```python
from build123d import *

# Parameters (mm, degrees)
SKETCH1_R           = 3.0607
BOSS_EXTRUDE1_DEPTH = 6.35
SKETCH2_R           = 8.20039
CUT_EXTRUDE1_DEPTH  = 7.35
BOSS_EXTRUDE2_DEPTH = 19.05
SKETCH4_R           = 8.20039
CUT_EXTRUDE2_DEPTH  = 19.05
CUT_EXTRUDE2_TAPER  = -12
SKETCH5_R           = 1.5875
CUT_EXTRUDE3_DEPTH  = 7.35
BOSS_EXTRUDE3_DEPTH = 6.35


with BuildPart() as part:
    # Sketch1 → Boss-Extrude1 (new body)
    with BuildSketch(Plane(origin=(0, 91.487983019, 0), x_dir=(1, 0, 0), z_dir=(0, 1, 0))):
        with BuildLine():
            Line((-19.645108088, -156.928503968), (88.304891912, -156.928503968))
            ThreePointArc((88.304891912, -156.928503968), (95.040084003, -154.138696059), (97.829891912, -147.403503968))
            Line((97.829891912, -147.403503968), (97.829891912, -64.853503968))
            ThreePointArc((97.829891912, -64.853503968), (95.040084003, -58.118311877), (88.304891912, -55.328503968))
            Line((88.304891912, -55.328503968), (-19.645108088, -55.328503968))
            ThreePointArc((-19.645108088, -55.328503968), (-26.380300179, -58.118311877), (-29.170108088, -64.853503968))
            Line((-29.170108088, -64.853503968), (-29.170108088, -147.403503968))
            ThreePointArc((-29.170108088, -147.403503968), (-26.380300179, -154.138696059), (-19.645108088, -156.928503968))
        make_face()
        with Locations((-23.740858088, -151.499253968)):
            Circle(SKETCH1_R, mode=Mode.SUBTRACT)
        with Locations((-23.740858088, -60.757753968)):
            Circle(SKETCH1_R, mode=Mode.SUBTRACT)
        with Locations((92.400641912, -60.757753968)):
            Circle(SKETCH1_R, mode=Mode.SUBTRACT)
        with Locations((92.400641912, -151.499253968)):
            Circle(SKETCH1_R, mode=Mode.SUBTRACT)
    extrude(amount=BOSS_EXTRUDE1_DEPTH)

    # Sketch2 → Cut-Extrude1 (cut, through all)
    with BuildSketch(Plane.XZ.offset(-91.487983019)):
        with Locations((47.029891912, 106.128503968)):
            Circle(SKETCH2_R)
        with Locations((21.629891912, 106.128503968)):
            Circle(SKETCH2_R)
    extrude(amount=-CUT_EXTRUDE1_DEPTH, mode=Mode.SUBTRACT)

    # Sketch3 → Boss-Extrude2 (add)
    with BuildSketch(Plane(origin=(0, 97.837983019, 0), x_dir=(1, 0, 0), z_dir=(0, 1, 0))):
        with BuildLine():
            Line((21.629891912, -88.983503968), (47.029891912, -88.983503968))
            ThreePointArc((47.029891912, -88.983503968), (64.174891912, -106.128503968), (47.029891912, -123.273503968))
            Line((47.029891912, -123.273503968), (21.629891912, -123.273503968))
            ThreePointArc((21.629891912, -123.273503968), (4.484891912, -106.128503968), (21.629891912, -88.983503968))
        make_face()
    extrude(amount=BOSS_EXTRUDE2_DEPTH)

    # Sketch4 → Cut-Extrude2 (cut)
    with BuildSketch(Plane.XZ.offset(-97.837983019)):
        with Locations((21.629891912, 106.128503968)):
            Circle(SKETCH4_R)
        with Locations((47.029891912, 106.128503968)):
            Circle(SKETCH4_R)
    extrude(amount=-CUT_EXTRUDE2_DEPTH, taper=CUT_EXTRUDE2_TAPER, mode=Mode.SUBTRACT)

    # Sketch5 → Cut-Extrude3 (cut, through all)
    with BuildSketch(Plane(origin=(0, 97.837983019, 0), x_dir=(1, 0, 0), z_dir=(0, 1, 0))):
        with Locations((73.223641912, -111.526003968)):
            Circle(SKETCH5_R)
        with Locations((73.223641912, -101.874003968)):
            Circle(SKETCH5_R)
        with Locations((73.223641912, -92.222003968)):
            Circle(SKETCH5_R)
    extrude(amount=-CUT_EXTRUDE3_DEPTH, mode=Mode.SUBTRACT)

    # Sketch6 → Boss-Extrude3 (add)
    with BuildSketch(Plane(origin=(0, 97.837983019, 0), x_dir=(1, 0, 0), z_dir=(0, 1, 0))):
        with BuildLine():
            Line((-32.345108088, -64.853503968), (-32.345108088, -147.403503968))
            ThreePointArc((-32.345108088, -147.403503968), (-28.625364209, -156.383760089), (-19.645108088, -160.103503968))
            Line((-19.645108088, -160.103503968), (88.304891912, -160.103503968))
            ThreePointArc((88.304891912, -160.103503968), (97.285148033, -156.383760089), (101.004891912, -147.403503968))
            Line((101.004891912, -147.403503968), (101.004891912, -64.853503968))
            ThreePointArc((101.004891912, -64.853503968), (97.285148033, -55.873247847), (88.304891912, -52.153503968))
            Line((88.304891912, -52.153503968), (-19.645108088, -52.153503968))
            ThreePointArc((-19.645108088, -52.153503968), (-28.625364209, -55.873247847), (-32.345108088, -64.853503968))
        make_face()
        with BuildLine():
            Line((-19.645108088, -156.928503968), (88.304891912, -156.928503968))
            ThreePointArc((88.304891912, -156.928503968), (95.040084003, -154.138696059), (97.829891912, -147.403503968))
            Line((97.829891912, -147.403503968), (97.829891912, -64.853503968))
            ThreePointArc((97.829891912, -64.853503968), (95.040084003, -58.118311877), (88.304891912, -55.328503968))
            Line((88.304891912, -55.328503968), (-19.645108088, -55.328503968))
            ThreePointArc((-19.645108088, -55.328503968), (-26.380300179, -58.118311877), (-29.170108088, -64.853503968))
            Line((-29.170108088, -64.853503968), (-29.170108088, -147.403503968))
            ThreePointArc((-29.170108088, -147.403503968), (-26.380300179, -154.138696059), (-19.645108088, -156.928503968))
        make_face(mode=Mode.SUBTRACT)
    extrude(amount=-BOSS_EXTRUDE3_DEPTH)


solid = part.part
```
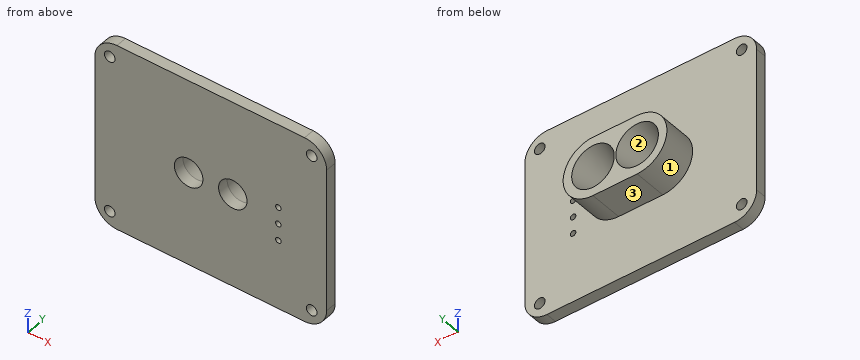
Read the model definition and answer for the solid it produces. Units are mm, in the model's axes. Face numbers are marked on the shaded views. Round coordinates to 2 decimals unless told otherwise and drop trailing zeros. Loops run counter-clockwise (first coordinate to the right, second up) from the corner with the lowest first, then second, coordinate; pieces in that order, holes last. Notation, with made-up numbers: (66, 30.5) -> (113, 30.5) arc R19 ccw to (113, 40.5) -> close; hole circle Ø4 at (-7.5, 64.5). An arc over 180 degrees is marked (long way). One line per item, written item: value.
1) A cutting plane is placed at C-C (y = 105.25). Determine the outline of the cut face in (x, z) (1 decimal).
Answer list:
outline: (21.6, 89) -> (47, 89) arc R17.1 ccw to (47, 123.3) -> (21.6, 123.3) arc R17.1 ccw to start; hole circle Ø19.6 at (21.6, 106.1); hole circle Ø19.6 at (47, 106.1)
2) Flat-ended cylindrical pins translate along their axes: P1, Ø7, axis at x = -23.74, z = 60.76, coming from the -Y side; P2, Ø8, axis at x = 5, z = 67.5, coming from the +Y side; P3, Ø12, axis at x = 13.5, y = 104, coming from the +Z side; P4, Ø8, axis at y = 113.5, z = 112, coming from the +X side. Find the tip coordinate at first contact, or state that the pin passes through.
Answer list:
P1: stops at y = 91.49
P2: stops at y = 97.84
P3: stops at z = 123.14
P4: stops at x = 64.07
3) A cutting plane is placed at B-B (x = 62.5). Determine the outline of the cut face in (y, z).
Answer list:
outline: (91.49, 52.15) -> (97.84, 52.15) -> (97.84, 98.74) -> (116.89, 98.74) -> (116.89, 113.52) -> (97.84, 113.52) -> (97.84, 160.1) -> (91.49, 160.1) -> close
4) A cutting plane is placed at D-D (z = 120.5). Determine the outline of the cut face in (x, y), and give its area (3 significant figures).
Answer list:
outline: (-32.35, 91.49) -> (101, 91.49) -> (101, 97.84) -> (56.38, 97.84) -> (56.38, 116.89) -> (12.28, 116.89) -> (12.28, 97.84) -> (-32.35, 97.84) -> close
area: 1,690 mm²
5) A cutting plane is placed at A-A (y = 94). Give the number of separate pieces and of enclosed holes in the cut face, and give its area (3 significant figures).
Answer list:
separate pieces: 1
enclosed holes: 9
area: 13,700 mm²
6) The mould has two halves that part along X. Classify the marked faces 1, 2 and 3: pulls with the +X half, pulls with the -X half, needs draft (parallel to the pull), parting line crosses it, or undercut.
Answer list:
face 1: pulls with the -X half
face 2: undercut
face 3: needs draft
7) Consider L1, parallel to X at y = 94.75, z = 61.5; L2, parallel to X at y = 107, z = 98.5; L3, parallel to Z at x = 20, y = 110. Determine where each line is inside the solid, lowest interval first. Write a range as [from, to].
Answer list:
L1: x = [-31.89, -26.71], [-20.77, 89.43], [95.37, 100.55]
L2: x = [6.28, 14.94], [28.32, 40.34], [53.72, 62.38]
L3: z = [89.06, 95.47], [116.79, 123.2]
